```python
from build123d import *

# Parameters (mm, degrees)
SKICA1_R                 = 2
P_IDAT_VYSUNUT_M1_DEPTH  = 1
SKICA2_R                 = 1.15
ODEBRAT_VYSUNUT_M1_DEPTH = 2
SKICA3_R                 = 3
SKICA3_R_2               = 2
P_IDAT_VYSUNUT_M2_DEPTH  = 3
ODEBRAT_VYSUNUT_M2_DEPTH = 10


with BuildPart() as part:
    # Skica1 → Přidat vysunutím1 (new body)
    with BuildSketch(Plane(origin=(0, 0, 0), x_dir=(1, 0, 0), z_dir=(0, 1, 0))):
        with BuildLine():
            Line((-12.62, 1.495192295), (-2.5, 2.307395517))
            Line((-2.5, 2.307395517), (-2.5, 5.25))
            ThreePointArc((-2.5, 5.25), (0, 7.75), (2.5, 5.25))
            Line((2.5, 5.25), (2.5, 2.307395517))
            Line((2.5, 2.307395517), (12.62, 1.495192295))
            ThreePointArc((12.62, 1.495192295), (14, 0), (12.62, -1.495192295))
            Line((12.62, -1.495192295), (2.5, -2.307395517))
            Line((2.5, -2.307395517), (2.5, -5.25))
            ThreePointArc((2.5, -5.25), (0, -7.75), (-2.5, -5.25))
            Line((-2.5, -5.25), (-2.5, -2.307395517))
            Line((-2.5, -2.307395517), (-12.62, -1.495192295))
            ThreePointArc((-12.62, -1.495192295), (-14, 0), (-12.62, 1.495192295))
        make_face()
        Circle(SKICA1_R, mode=Mode.SUBTRACT)
    extrude(amount=P_IDAT_VYSUNUT_M1_DEPTH)

    # Skica2 → Odebrat vysunutím1 (cut)
    with BuildSketch(Plane(origin=(0, 1, 0), x_dir=(1, 0, 0), z_dir=(0, 1, 0))):
        with Locations((-8.5, 0)):
            Circle(SKICA2_R)
        with Locations((8.5, 0)):
            Circle(SKICA2_R)
    extrude(amount=-ODEBRAT_VYSUNUT_M1_DEPTH, mode=Mode.SUBTRACT)

    # Skica3 → Přidat vysunutím2 (add)
    with BuildSketch(Plane(origin=(0, 1, 0), x_dir=(1, 0, 0), z_dir=(0, 1, 0))):
        Circle(SKICA3_R)
        Circle(SKICA3_R_2, mode=Mode.SUBTRACT)
    extrude(amount=P_IDAT_VYSUNUT_M2_DEPTH)

    # Skica4 → Odebrat vysunutím2 (cut)
    with BuildSketch(Plane.XZ):
        with BuildLine():
            Line((-2.5, 2.307395517), (-2.5, 10.588101579))
            Line((-2.5, 10.588101579), (18.005147354, 10.588101579))
            Line((18.005147354, 10.588101579), (18.005147354, -8.717716122))
            Line((18.005147354, -8.717716122), (-2.5, -8.868206906))
            Line((-2.5, -8.868206906), (-2.5, -2.307395517))
            ThreePointArc((-2.5, -2.307395517), (3.402069087, 0), (-2.5, 2.307395517))
        make_face()
    extrude(amount=-ODEBRAT_VYSUNUT_M2_DEPTH, mode=Mode.SUBTRACT)


solid = part.part
```
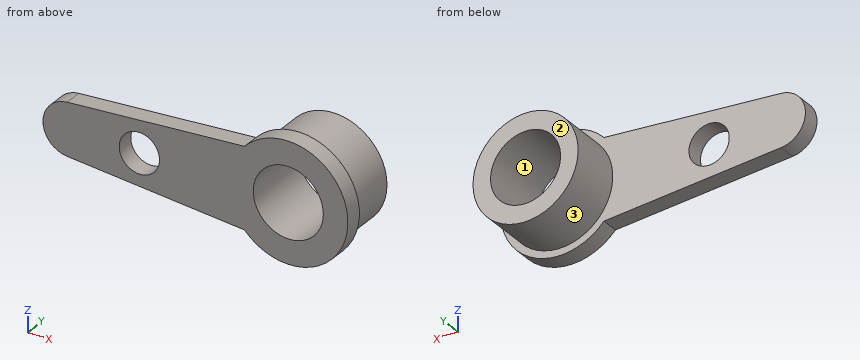
CAD build for the part. Positions are in the model's coordinates, mm. Face numbers are marked on the shaded views. Round coordinates to 2 decimals unless told otherwise and drop trailing zeros. Order: outer loops, then holes, each group sorted by start corner. A loop starts at its lowest first (then second) coordinate and runs counter-clockwise, first axis right, second up.
Item 1: Pin check, flat tips, straight feed: pin 1 (2 mm diameter, centred on y = 1.5, z = 1.5, fed in from +X); pin 2 (4 mm diameter, centred on x = -9.5, z = -1.5, fed in from +Y); pin 3 (2 mm diameter, centred on x = -8.5, z = 0, fed in from -Y); pin 4 (4 mm diameter, centred on x = -3.5, z = -1.5, fed in from -Y). Stop position of each tip, or through.
Item 2: Probe line 1 along Z through (x, y) = (0, 1.4); line 2 along Y through (x, z) = (-4.25, 0). List the from-to ranges inside material, lowest first.
Item 3: Saw through at B-B on z = 0. Write the cut outline in (x, y), then the cut area to 3 significant figures.
Item 4: Saw through at D-D on x = -8.5. Write the cut outline in (y, z), then the cut area to 3 significant figures.
Item 5: Mould opens along Z. For the marked faces 1, 2 and 3 say: pulls with the +Z half, pulls with the -Z half, needs draft (parallel to the pull), parting line crosses it, or undercut.
Item 6: Saw through at C-C on y = 3.15. Write the cut outline in (x, z).
Item 7: Saw through at A-A on x = 0. Write the cut outline in (y, z).
Reported:
1. pin 1: stops at x = 3.34
1. pin 2: stops at y = 1
1. pin 3: passes through
1. pin 4: stops at y = 0
2. line 1: z = -3 to -2, 2 to 3
2. line 2: y = 0 to 1
3. outline: (-14, 0) - (-9.65, 0) - (-9.65, 1) - (-14, 1) - close; (-7.35, 0) - (-2, 0) - (-2, 4) - (-3, 4) - (-3, 1) - (-7.35, 1) - close; (2, 0) - (3.4, 0) - (3.4, 1) - (3, 1) - (3, 4) - (2, 4) - close
3. area: 17.1 mm2
4. outline: (0, -1.83) - (1, -1.83) - (1, -1.15) - (0, -1.15) - close; (0, 1.15) - (1, 1.15) - (1, 1.83) - (0, 1.83) - close
4. area: 1.35 mm2
5. face 1: undercut
5. face 2: needs draft
5. face 3: parting line crosses it
6. outline: circle Ø6 at (0, 0); hole circle Ø4 at (0, 0)
7. outline: (0, -3.4) - (1, -3.4) - (1, -3) - (4, -3) - (4, -2) - (0, -2) - close; (0, 2) - (4, 2) - (4, 3) - (1, 3) - (1, 3.4) - (0, 3.4) - close
